Build history of the part. All positions in model axes, mm. Round coordinates to 2 decimals unless told otherwise and drop trailing zeros. Loops run counter-clockwise (first coordinate to the right, second up) from the corner with the lowest first, then second, coordinate; pieces in that order, holes last. Notation, with made-up numbers: M -0.5,73 L 29.5,73 A7 ccw 29.5,82 Z; hole C -25.5,-21 d10. An arc over 180 degrees is marked long. Use one line per item in the form item = value. Start each with the question number.
```python
from build123d import *

# Parameters (mm, degrees)
BOSS_EXTRUDE1_DEPTH      = 6
M3_CLEARANCE_HOLE1_D     = 3.6
M3_CLEARANCE_HOLE1_DEPTH = 6
M3_CLEARANCE_HOLE1_TIP   = 1.081549114
FILLET1_R                = 15
SKETCH4_W                = 65
SKETCH4_H                = 9
SKETCH4_W_2              = 32.5
CUT_EXTRUDE1_DEPTH       = 2
M4_CLEARANCE_HOLE1_D     = 4.8
M4_CLEARANCE_HOLE1_DEPTH = 6
M4_CLEARANCE_HOLE1_TIP   = 1.442065486
CHAMFER1_SIZE            = 2.4


with BuildPart() as part:
    # Sketch1 → Boss-Extrude1 (new body)
    with BuildSketch(Plane.XY):
        with BuildLine():
            Line((-32.5, 95), (-32.5, -95))
            ThreePointArc((-32.5, -95), (0, -62.5), (32.5, -95))
            Line((32.5, -95), (32.5, 95))
            Line((32.5, 95), (-32.5, 95))
        make_face()
        with BuildLine():
            ThreePointArc((32.5, -95), (0, -62.5), (-32.5, -95))
            Line((-32.5, -95), (-15.5, -95))
            Line((-15.5, -95), (-15.5, -79.5))
            Line((-15.5, -79.5), (15.5, -79.5))
            Line((15.5, -79.5), (15.5, -95))
            Line((15.5, -95), (32.5, -95))
        make_face()
        with BuildLine():
            Line((-15.5, -95), (-32.5, -95))
            ThreePointArc((-32.5, -95), (0, -127.5), (32.5, -95))
            Line((32.5, -95), (15.5, -95))
            Line((15.5, -95), (15.5, -110.5))
            Line((15.5, -110.5), (-15.5, -110.5))
            Line((-15.5, -110.5), (-15.5, -95))
        make_face()
        with BuildLine():
            Line((-14, -95), (-15.5, -95))
            Line((-15.5, -95), (-15.5, -110.5))
            Line((-15.5, -110.5), (15.5, -110.5))
            Line((15.5, -110.5), (15.5, -95))
            Line((15.5, -95), (14, -95))
            ThreePointArc((14, -95), (0, -109), (-14, -95))
        make_face()
        with BuildLine():
            Line((-15.5, -79.5), (-15.5, -95))
            Line((-15.5, -95), (-14, -95))
            ThreePointArc((-14, -95), (0, -81), (14, -95))
            Line((14, -95), (15.5, -95))
            Line((15.5, -95), (15.5, -79.5))
            Line((15.5, -79.5), (-15.5, -79.5))
        make_face()
    extrude(amount=BOSS_EXTRUDE1_DEPTH)

    # M3 Clearance Hole1
    with Locations(Plane(origin=(0, 0, 0), x_dir=(-1, 0, 0), z_dir=(0, 0, -1))):
        with Locations((-15.5, -110.5), (15.5, -110.5), (15.5, -79.5), (-15.5, -79.5)):
            Hole(M3_CLEARANCE_HOLE1_D / 2, depth=M3_CLEARANCE_HOLE1_DEPTH)
            with Locations((0, 0, -(M3_CLEARANCE_HOLE1_DEPTH + M3_CLEARANCE_HOLE1_TIP / 2))):  # 118° drill point
                Cone(0, M3_CLEARANCE_HOLE1_D / 2, M3_CLEARANCE_HOLE1_TIP, mode=Mode.SUBTRACT)

    # Fillet1
    fillet1_edges = [part.edges().sort_by_distance(p)[0] for p in [
        (-32.5, 95, 3),
        (32.5, 95, 3),
    ]]
    fillet(fillet1_edges, radius=FILLET1_R)

    # Sketch4 → Cut-Extrude1 (cut)
    with BuildSketch(Plane.XY.offset(6)):
        with Locations((0, 75.5)):
            Rectangle(SKETCH4_W, SKETCH4_H)
        with Locations((-16.25, 7.5)):
            Rectangle(SKETCH4_W_2, SKETCH4_H)
        with Locations((16.25, 7.5)):
            Rectangle(SKETCH4_W_2, SKETCH4_H)
        with Locations((0, -60.5)):
            Rectangle(SKETCH4_W, SKETCH4_H)
    extrude(amount=-CUT_EXTRUDE1_DEPTH, mode=Mode.SUBTRACT)

    # M4 Clearance Hole1
    with Locations(Plane.XY.offset(4)):
        with Locations((-24.5, -60.5), (-24.5, 75.5), (24.5, 75.5), (0, 75.5), (-24.5, 7.5), (0, 7.5), (24.5, 7.5), (24.5, -60.5), (0, -60.5)):
            Hole(M4_CLEARANCE_HOLE1_D / 2, depth=M4_CLEARANCE_HOLE1_DEPTH)
            with Locations((0, 0, -(M4_CLEARANCE_HOLE1_DEPTH + M4_CLEARANCE_HOLE1_TIP / 2))):  # 118° drill point
                Cone(0, M4_CLEARANCE_HOLE1_D / 2, M4_CLEARANCE_HOLE1_TIP, mode=Mode.SUBTRACT)

    # Chamfer1
    chamfer1_edges = [part.edges().sort_by_distance(p)[0] for p in [
        (-22.1, -60.5, 0),
        (2.4, -60.5, 0),
        (26.9, -60.5, 0),
        (26.9, 7.5, 0),
        (2.4, 7.5, 0),
        (-22.1, 7.5, 0),
        (2.4, 75.5, 0),
        (26.9, 75.5, 0),
        (-22.1, 75.5, 0),
        (13.7, -79.5, 0),
        (-17.3, -79.5, 0),
        (-17.3, -110.5, 0),
        (13.7, -110.5, 0),
    ]]
    chamfer(chamfer1_edges, length=CHAMFER1_SIZE)


solid = part.part
```
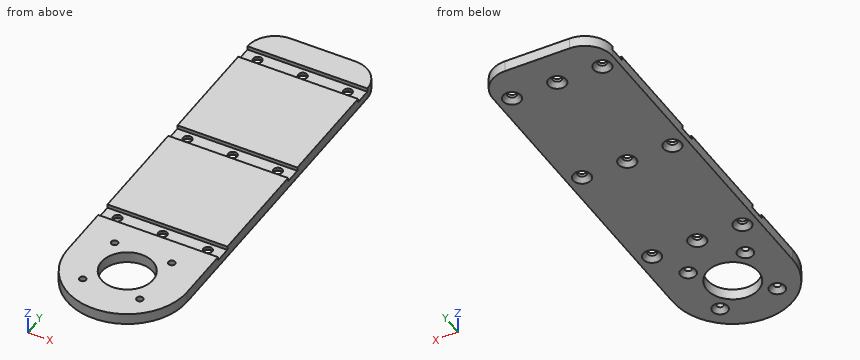
Q1. Wall check: probe 1 along X at (y, z) = (-79.5, 5.1); probe 2 along Y at (x, z) = (24.5, 2.85); probe 3 along X at (y, z) = (-61, 2.3). Give the ranges that are in metal, low to high.
Q2. Drop flat-ended pins along their axis: P1, Ø1, axis at x = -4, z = 4.5, coming from the -Y side; P2, Ø6, axis at x = 0, y = 75.5, coming from the -Z side; P3, Ø2.5, axis at x = -1.5, y = -59, coming from the +Z side; P4, Ø4.5, axis at x = 0, y = 7.5, coming from the +Z side. Give the stop position or say it passes through.
Q3. Saw through at B-B (y = -60.5). Give the cut face in (x, z), and give its area (3 significant figures).
Q4. Saw through at A-A (z = 5). Give the number of separate pieces and of enclosed holes in the cut face, and give its area (3 significant figures).
Filled in:
q1.probe_1 = -32.5 to -17.3, -13.7 to 13.7, 17.3 to 32.5
q1.probe_2 = -116.35 to -62.9, -58.1 to 5.1, 9.9 to 73.1, 77.9 to 93.27
q1.probe_3 = -32.5 to -26.95, -22.05 to -2.45, 2.45 to 22.05, 26.95 to 32.5
q2.P1 = -127.31
q2.P2 = 1.8
q2.P3 = 4
q2.P4 = through
q3.outline = M -32.5,0 L -29.3,0 L -26.9,2.4 L -26.9,4 L -32.5,4 Z; M -22.1,2.4 L -19.7,0 L -4.8,0 L -2.4,2.4 L -2.4,4 L -22.1,4 Z; M 2.4,2.4 L 4.8,0 L 19.7,0 L 22.1,2.4 L 22.1,4 L 2.4,4 Z; M 26.9,2.4 L 29.3,0 L 32.5,0 L 32.5,4 L 26.9,4 Z
q3.area = 185 mm²
q4.separate_pieces = 4
q4.enclosed_holes = 5
q4.area = 11,500 mm²
